Study the drawing (mm; zero at the part's minimum x, y, z) and answer. A direction names the side the tool comes from. Give positions to 0.01 mm unless a question says otherwise; leave off trailing zeros. Order: outer loops, then holes, each group sorted by start corner. A loop starts at its lowest first (then second) coordinate and runs counter-clockwise, first axis right, second up. Notation, with made-up numbers: (-12.75, 34.5) - (3.25, 34.5) arc R5 cw to (3.25, 42.5) - close; hole circle Ø11 at (55.5, 56). An arc over 180 degrees is marked (long way). Put each result on its own line as item: value.
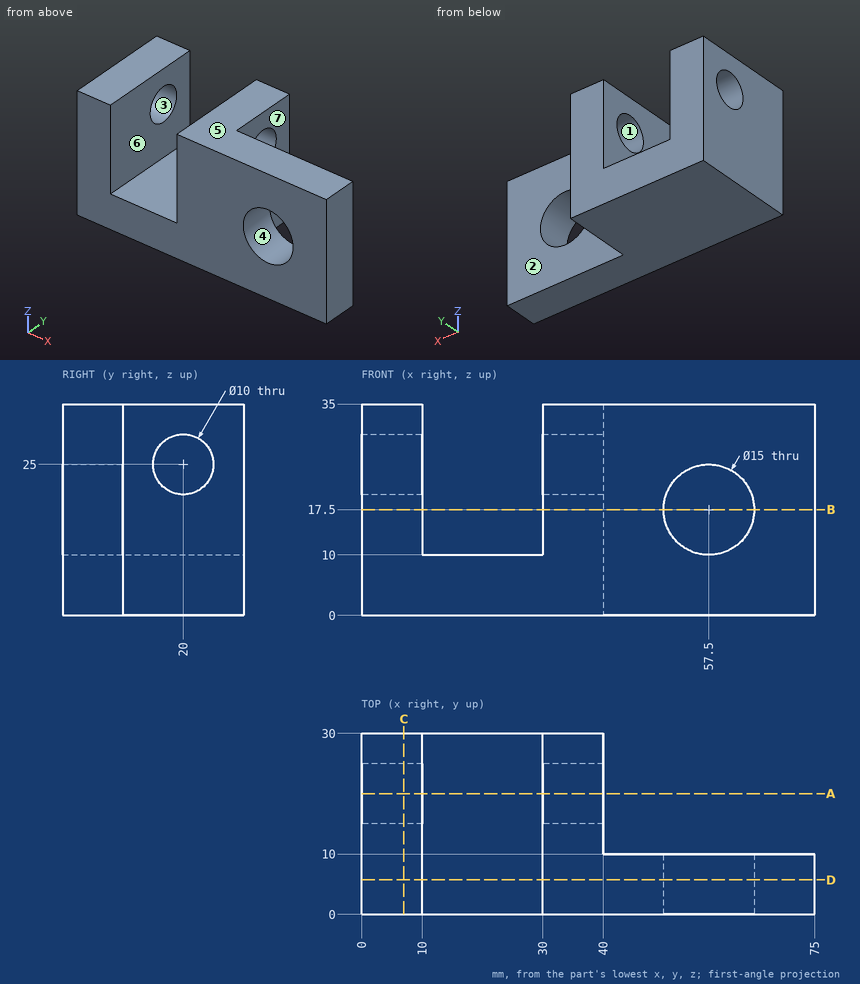
(1) Determine the mould class of the marked faces 1, 2, 3 and 4 for opening direction Y: pulls with the +Y half, pulls with the -Y half, needs draft (parallel to the pull), parting line crosses it, or undercut.
Geometry check:
face 1: undercut
face 2: pulls with the +Y half
face 3: undercut
face 4: needs draft
(2) Section C-C, the plane x = 7 is taken. Write down the section's boundary in (y, z), then the cut area to 3 significant figures.
Geometry check:
outline: (0, 0) - (30, 0) - (30, 35) - (0, 35) - close; hole circle Ø10 at (20, 25)
area: 971 mm²
(3) Section A-A, the plane y = 20 is taken. Write down the section's boundary in (x, z).
Geometry check:
outline: (0, 0) - (40, 0) - (40, 20) - (30, 20) - (30, 10) - (10, 10) - (10, 20) - (0, 20) - close; (0, 30) - (10, 30) - (10, 35) - (0, 35) - close; (30, 30) - (40, 30) - (40, 35) - (30, 35) - close
(4) Section D-D, the plane y = 5.75 is taken. Write down the section's boundary in (x, z), then the cut area to 3 significant figures.
Geometry check:
outline: (0, 0) - (75, 0) - (75, 35) - (30, 35) - (30, 10) - (10, 10) - (10, 35) - (0, 35) - close; hole circle Ø15 at (57.5, 17.5)
area: 1,950 mm²
(5) A tool of negligible diameter and unlimited length cuts with its end or side. For the marked faces 5, 6 and 7, from which of +Z, -Z, +X, -X, +Y, -Y can it reach the whole face along a straight path? Write none if from no direction.
Geometry check:
face 5: +Z, +X, -X, +Y, -Y
face 6: +Z, +Y, -Y
face 7: +Z, -Z, +X, +Y
(6) Straight lines are drawn through the part: line 1 (Y direction, x = 38, z = 25); line 2 (X direction, y = 26.5, z = 23.5); line 3 (Z direction, x = 11.5, y = 20.25). For each, find the intervals that lie inside material, in ascending order.
Geometry check:
line 1: y = 0 to 15, 25 to 30
line 2: x = 0 to 10, 30 to 40
line 3: z = 0 to 10
(7) Given pin 1 (8 mm diameter, centred on x = 44.5, z = 12.5, fed in from -Y); pin 2 (6 mm diameter, centred on y = 20, z = 25, fed in from -X); pin 3 (13 mm diameter, centred on y = 20, z = 25, fed in from +X), each flat-ended and moving along its own axis, determine where each tip first touches the part or whether it passes through.
Geometry check:
pin 1: stops at y = 0
pin 2: passes through
pin 3: stops at x = 40
(8) Section B-B, the plane z = 17.5 is taken. Write down the section's boundary in (x, y).
Geometry check:
outline: (0, 0) - (10, 0) - (10, 30) - (0, 30) - close; (30, 0) - (50, 0) - (50, 10) - (40, 10) - (40, 30) - (30, 30) - close; (65, 0) - (75, 0) - (75, 10) - (65, 10) - close
